Design review of the part shown in the three views and the two pictorial views. Dimensions are in mm from the part's minimum x, y and z. A direction names the side the tool comes from. Give positions to 0.01 mm unless a question says otherwise; leave off trailing zeros. Order: outer loops, then holes, each group sorted by start corner. A loop starts at its lowest first (then second) coordinate and runs counter-clockwise, first axis right, second up.
Item 1: Consider section D-D (z = 23). Give the boundary of the cut face in (x, y).
Item 2: Consider section A-A (x = 47). Give the boundary of the cut face in (y, z), plus the area to 3 significant figures.
Item 3: Consider section B-B (y = 14). Give the boundary of the cut face in (x, z).
Item 4: Consider section C-C (x = 18). Give the boundary of the cut face in (y, z), plus the area to 3 significant figures.
Item 5: For probe 1 along Y at (x, z) = (58, 20.25); probe 2 along Z at (x, y) = (40, 26.95); probe 3 along X at (y, z) = (26.25, 12.5), list the stretches that pass through material, from the lowest coordinate up.
Item 6: For P1, Ø2.5, axis at y = 14, z = 12.5, coming from the -X side; P2, Ø3.5, axis at x = 40, z = 12.5, coming from the +Y side; P3, Ø2, axis at y = 9.5, z = 12.5, coming from the -X side, all flat-tipped, find the tip position at first contact; note any pin that passes through.
Item 7: The part is to be moulded in two halves that separate along Y. For the marked faces 1, 2 and 3, say which applies: released by +Y, released by -Y, zero draft, split by the parting line, or undercut.
Item 8: Machinability: for the marked faces 4 and 5, which of the approach directions +Z, -Z, +X, -X, +Y, -Y give a long, thin tool a straight path to every point of the face, cutting with its end or side? Answer none if there is none.
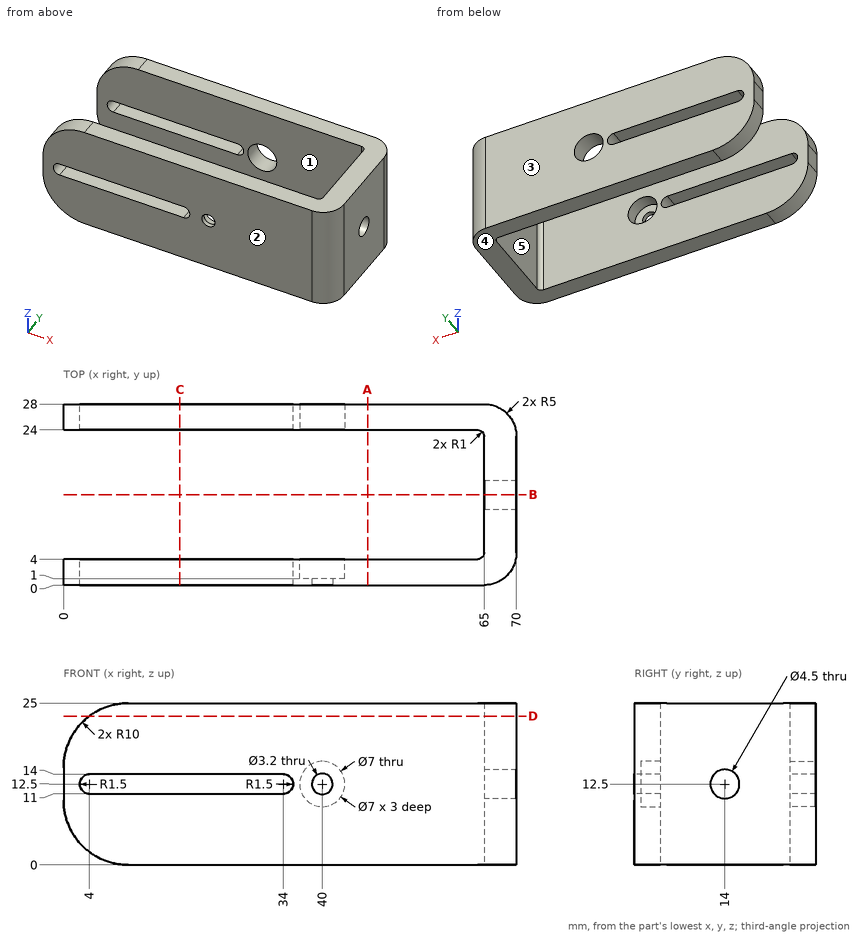
Resolved:
1. outline: (4, 0) - (65, 0) arc R5 ccw to (70, 5) - (70, 23) arc R5 ccw to (65, 28) - (4, 28) - (4, 24) - (64, 24) arc R1 cw to (65, 23) - (65, 5) arc R1 cw to (64, 4) - (4, 4) - close
2. outline: (0, 0) - (4, 0) - (4, 25) - (0, 25) - close; (24, 0) - (28, 0) - (28, 25) - (24, 25) - close
2. area: 200 mm2
3. outline: (65, 0) - (70, 0) - (70, 10.25) - (65, 10.25) - close; (65, 14.75) - (70, 14.75) - (70, 25) - (65, 25) - close
4. outline: (0, 0) - (4, 0) - (4, 11) - (0, 11) - close; (0, 14) - (4, 14) - (4, 25) - (0, 25) - close; (24, 0) - (28, 0) - (28, 11) - (24, 11) - close; (24, 14) - (28, 14) - (28, 25) - (24, 25) - close
4. area: 176 mm2
5. probe 1: y = 0 to 4, 24 to 28
5. probe 2: z = 0 to 9, 16 to 25
5. probe 3: x = 0 to 2.5, 35.5 to 36.5, 43.5 to 68.8
6. P1: passes through
6. P2: stops at y = 1
6. P3: stops at x = 65
7. face 1: undercut
7. face 2: released by -Y
7. face 3: released by +Y
8. face 4: -Z, +X, -X, +Y, -Y
8. face 5: +Z, -Z, -X
